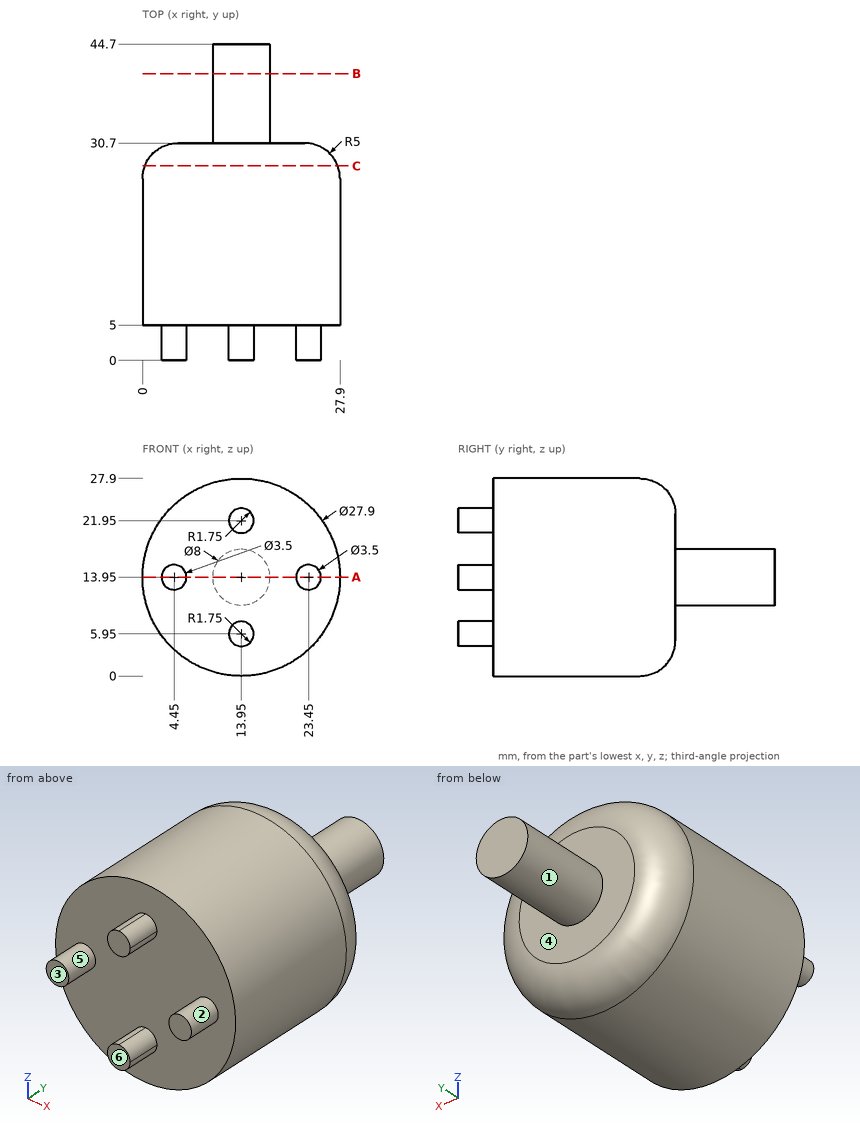
Part print with two shaded views. Sizes in mm from the minimum x, y, z corner. A direction names the side the tool comes from. Give positions to 0.01 mm unless a question says otherwise; leave off trailing zeros. Write each loop counter-clockwise with the first axis right and the second up, starting at its lowest first coordinate (ties: lowest second). Pieces come first, ordered by that corner, then holes.
1) Probe L1, parallel to Y at x = 8.25, z = 10.5; L2, parallel to Y at x = 14.5, z = 21; L3, parallel to Z at x = 11, y = 23. List the from-to ranges inside material, lowest first.
Resolved:
L1: y = 5 to 30.7
L2: y = 0 to 30.7
L3: z = 0.32 to 27.58
2) Cut at A-A on z = 13.95. Write the cut outline in (x, y), then the cut area to 3 significant figures.
Resolved:
outline: (0, 5) - (2.7, 5) - (2.7, 0) - (6.2, 0) - (6.2, 5) - (21.7, 5) - (21.7, 0) - (25.2, 0) - (25.2, 5) - (27.9, 5) - (27.9, 25.7) arc R5 ccw to (22.9, 30.7) - (17.95, 30.7) - (17.95, 44.7) - (9.95, 44.7) - (9.95, 30.7) - (5, 30.7) arc R5 ccw to (0, 25.7) - close
area: 853 mm2
3) Two-plate mould, pull along X, no slides. Class the marked faces 1, 2 and 3: released by +X, released by -X, zero draft, split by the parting line, or undercut.
Resolved:
face 1: split by the parting line
face 2: undercut
face 3: zero draft
4) Pin check, flat tips, straight feed: pin 1 (1.5 mm diameter, centred on x = 7, y = 21.5, fed in from -Z); pin 2 (4 mm diameter, centred on y = 23, z = 20, fed in from +X); pin 3 (1 mm diameter, centred on y = 12, z = 13, fed in from +X); pin 4 (4 mm diameter, centred on y = 36.5, z = 21.5, fed in from +X). Stop position of each tip, or through.
Resolved:
pin 1: stops at z = 1.45
pin 2: stops at x = 27.3
pin 3: stops at x = 27.89
pin 4: passes through
5) Cut at C-C on y = 27.5. Write the cut outline in (x, z).
Resolved:
outline: circle Ø27.23 at (13.95, 13.95)
6) Which spindle directions (+Z, -Z, +X, -X, +Y, -Y) get a long thin tool onto all of the face, cutting with end or side? Do the marked faces 4, 5 and 6. Say none if no direction does.
Resolved:
face 4: +Y
face 5: -Y
face 6: +Z, -Z, +X, -X, -Y
7) Cut at B-B on y = 40.5. Write the cut outline in (x, z), then the cut area to 3 significant figures.
Resolved:
outline: circle Ø8 at (13.95, 13.95)
area: 50.3 mm2
